For this review, take the finished solid that the model builds, in its own axes (mm). Face numbers are marked on the shaded views. Coordinates: 2 decimals unless noted, no trailing zeros. Loops run counter-clockwise (first coordinate to the right, second up) from the corner with the lowest first, then second, coordinate; pieces in that order, holes last. Notation, with made-up numbers: (78.5, 10) - (129.5, 10) arc R15 cw to (129.5, 22) - close; hole circle Ø7 at (27.5, -26.5). An arc over 180 degrees is marked (long way). One line per item, written item: value. Start each with the question number.
1. To check wall thickness, follow line 1 (Z direction, x = 157.5, y = 30.5) (3 decimals); line 2 (Z direction, x = 211, y = 21.5); line 3 (X direction, y = 26.5, z = -6). State the ranges of each line that lie inside material, in increasing order. Write a range as from..to.
2. The part is to be moulded in two halves that separate along X. For the marked faces 1, 2 and 3, say which applies: released by +X, released by -X, zero draft, split by the parting line, or undercut.
3. Take a section at C-C, the plane z = -21. State the section outline as (x, y) points, and give its area (3 significant figures).
4. Insertion check: pin 1 (12 mm diameter, centred on x = 223, y = 29.5, fed in from +Z); pin 2 (0.5 mm diameter, centred on y = 36.5, z = 1.5, fed in from +X); pin 3 (0.5 mm diameter, centred on y = 8, z = 1.5, fed in from -X). Each pin has a flat end and moves straight along its axis. Give the tip position at first contact, or say it passes through.
5. Take a section at B-B, the plane y = 15. State the section outline as (x, z) points (3 decimals).
6. Take a section at A-A, the plane x = 248. State the section outline as (y, z) points.
7. Take a section at D-D, the plane x = 177. State the section outline as (y, z) points (3 decimals).
```python
from build123d import *

# Parameters (mm, degrees)
BASE_FLANGE1_DEPTH = 44.45
SKETCH6_W          = 31.75
SKETCH6_H          = 3.429
CUT_EXTRUDE1_DEPTH = 284.468887342
SKETCH7_W          = 31.75
SKETCH7_H          = 3.429
CUT_EXTRUDE2_DEPTH = 272.141941158
FILLET1_R          = 12.7
CUT_EXTRUDE3_DEPTH = 284.468887342
CUT_EXTRUDE4_DEPTH = 272.141941158
SKETCH10_R         = 3.175
CUT_EXTRUDE5_DEPTH = 284.468887342


# Sheet-metal steps are written as plain solids
with BuildPart() as part:
    # Sketch1 → Base-Flange1 (new body)
    with BuildSketch(Plane(origin=(0, 0, 0), x_dir=(1, 0, 0), z_dir=(0, 1, 0))):
        with BuildLine():
            Line((0, 0), (193.606119446, 0))
            ThreePointArc((193.606119446, 0), (194.29331522, 0.075260177), (194.947932427, 0.297472776))
            Line((194.947932427, 0.297472776), (276.015713671, 38.1))
            Line((276.015713671, 38.1), (277.357526652, 35.222472776))
            Line((277.357526652, 35.222472776), (196.289745408, -2.580054448))
            ThreePointArc((196.289745408, -2.580054448), (194.980510995, -3.024479645), (193.606119446, -3.175))
            Line((193.606119446, -3.175), (0, -3.175))
            Line((0, -3.175), (0, 0))
        make_face()
    extrude(amount=BASE_FLANGE1_DEPTH)

    # Sketch6 → Cut-Extrude1 (cut, through all)
    with BuildSketch(Plane(origin=(0, 0, 0), x_dir=(-1, 0, 0), z_dir=(0, 0, -1))):
        with Locations((-136.525, 7.9375)):
            Rectangle(SKETCH6_W, SKETCH6_H)
        with Locations((-60.325, 36.5125)):
            Rectangle(SKETCH6_W, SKETCH6_H)
        with Locations((-136.525, 36.5125)):
            Rectangle(SKETCH6_W, SKETCH6_H)
        with Locations((-60.325, 7.9375)):
            Rectangle(SKETCH6_W, SKETCH6_H)
    extrude(amount=-CUT_EXTRUDE1_DEPTH, mode=Mode.SUBTRACT)

    # Sketch7 → Cut-Extrude2 (cut, through all)
    with BuildSketch(Plane(origin=(34.704969781, 0, 74.425047871), x_dir=(-0.9063077870366493, 0, 0.42261826174070083), z_dir=(-0.4226182617407009, 0, -0.9063077870366494))):
        with Locations((-228.156946417, 36.5125)):
            Rectangle(SKETCH7_W, SKETCH7_H)
        with Locations((-228.156946417, 7.9375)):
            Rectangle(SKETCH7_W, SKETCH7_H)
    extrude(amount=-CUT_EXTRUDE2_DEPTH, mode=Mode.SUBTRACT)

    # Fillet1
    fillet1_edges = [part.edges().sort_by_distance(p)[0] for p in [
        (0, 44.45, 1.5875),
        (0, 0, 1.5875),
        (276.686620162, 44.45, -36.661236388),
        (276.686620162, 0, -36.661236388),
    ]]
    fillet(fillet1_edges, radius=FILLET1_R)

    # Sketch8 → Cut-Extrude3 (cut, through all)
    with BuildSketch(Plane(origin=(0, 0, 0), x_dir=(-1, 0, 0), z_dir=(0, 0, -1))):
        with BuildLine():
            ThreePointArc((-44.938784585, 36.5125), (-46.030818439, 39.40175), (-47.122852293, 36.5125))
            ThreePointArc((-47.122852293, 36.5125), (-46.030818439, 33.62325), (-44.938784585, 36.5125))
        make_face()
        with BuildLine():
            ThreePointArc((-75.711215415, 36.5125), (-74.619181561, 33.62325), (-73.527147707, 36.5125))
            ThreePointArc((-73.527147707, 36.5125), (-74.619181561, 39.40175), (-75.711215415, 36.5125))
        make_face()
        with BuildLine():
            ThreePointArc((-121.138784585, 36.5125), (-122.230818439, 39.40175), (-123.322852293, 36.5125))
            ThreePointArc((-123.322852293, 36.5125), (-122.230818439, 33.62325), (-121.138784585, 36.5125))
        make_face()
        with BuildLine():
            ThreePointArc((-151.911215415, 36.5125), (-150.819181561, 33.62325), (-149.727147707, 36.5125))
            ThreePointArc((-149.727147707, 36.5125), (-150.819181561, 39.40175), (-151.911215415, 36.5125))
        make_face()
        with BuildLine():
            ThreePointArc((-151.911215415, 7.9375), (-150.819181561, 5.04825), (-149.727147707, 7.9375))
            ThreePointArc((-149.727147707, 7.9375), (-150.819181561, 10.82675), (-151.911215415, 7.9375))
        make_face()
        with BuildLine():
            ThreePointArc((-121.138784585, 7.9375), (-122.230818439, 10.82675), (-123.322852293, 7.9375))
            ThreePointArc((-123.322852293, 7.9375), (-122.230818439, 5.04825), (-121.138784585, 7.9375))
        make_face()
        with BuildLine():
            ThreePointArc((-75.711215415, 7.9375), (-74.619181561, 5.04825), (-73.527147707, 7.9375))
            ThreePointArc((-73.527147707, 7.9375), (-74.619181561, 10.82675), (-75.711215415, 7.9375))
        make_face()
        with BuildLine():
            ThreePointArc((-44.938784585, 7.9375), (-46.030818439, 10.82675), (-47.122852293, 7.9375))
            ThreePointArc((-47.122852293, 7.9375), (-46.030818439, 5.04825), (-44.938784585, 7.9375))
        make_face()
    extrude(amount=-CUT_EXTRUDE3_DEPTH, mode=Mode.SUBTRACT)

    # Sketch9 → Cut-Extrude4 (cut, through all)
    with BuildSketch(Plane(origin=(34.704969781, 0, 74.425047871), x_dir=(-0.9063077870366492, 0, 0.42261826174070116), z_dir=(-0.42261826174070116, 0, -0.9063077870366492))):
        with BuildLine():
            ThreePointArc((-214.95479871, 36.5125), (-213.862764856, 33.62325), (-212.770731003, 36.5125))
            ThreePointArc((-212.770731003, 36.5125), (-213.862764856, 39.40175), (-214.95479871, 36.5125))
        make_face()
        with BuildLine():
            ThreePointArc((-241.359094124, 36.5125), (-242.451127978, 39.40175), (-243.543161832, 36.5125))
            ThreePointArc((-243.543161832, 36.5125), (-242.451127978, 33.62325), (-241.359094124, 36.5125))
        make_face()
        with BuildLine():
            ThreePointArc((-241.359094124, 7.9375), (-242.451127978, 10.82675), (-243.543161832, 7.9375))
            ThreePointArc((-243.543161832, 7.9375), (-242.451127978, 5.04825), (-241.359094124, 7.9375))
        make_face()
        with BuildLine():
            ThreePointArc((-214.95479871, 7.9375), (-213.862764856, 5.04825), (-212.770731003, 7.9375))
            ThreePointArc((-212.770731003, 7.9375), (-213.862764856, 10.82675), (-214.95479871, 7.9375))
        make_face()
    extrude(amount=-CUT_EXTRUDE4_DEPTH, mode=Mode.SUBTRACT)

    # Sketch10 → Cut-Extrude5 (cut, through all)
    with BuildSketch(Plane(origin=(0, 0, 0), x_dir=(-1, 0, 0), z_dir=(0, 0, -1))):
        with Locations((-65.0875, 22.225)):
            Circle(SKETCH10_R)
    extrude(amount=-CUT_EXTRUDE5_DEPTH, mode=Mode.SUBTRACT)


solid = part.part
```
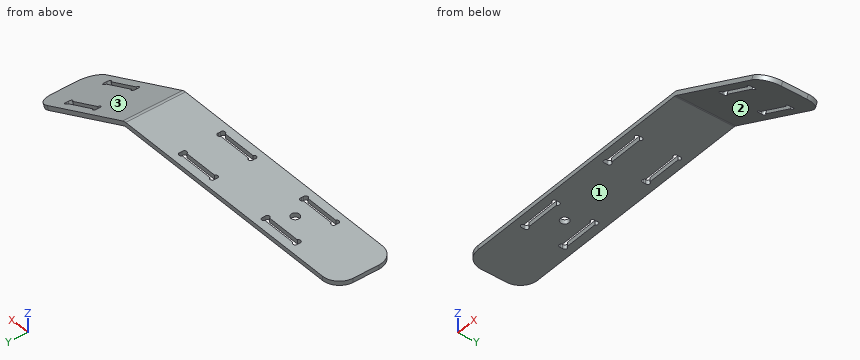
Solutions:
1. line 1: 0..3.175
1. line 2: -7.78..-4.28
1. line 3: 207.18..214.69
2. face 1: zero draft
2. face 2: released by -X
2. face 3: released by +X
3. outline: (239.34, 0) - (246.86, 0) - (246.86, 6.22) - (239.34, 6.22) - close; (239.34, 9.65) - (246.86, 9.65) - (246.86, 34.8) - (239.34, 34.8) - close; (239.34, 38.23) - (246.86, 38.23) - (246.86, 44.45) - (239.34, 44.45) - close
3. area: 282 mm2
4. pin 1: z = -7.08
4. pin 2: x = 199.14
4. pin 3: x = 0.81
5. outline: (0, 0) - (193.606, 0) arc R3.175 cw to (194.948, -0.297) - (276.016, -38.1) - (277.358, -35.222) - (196.29, 2.58) arc R6.35 ccw to (193.606, 3.175) - (0, 3.175) - close
6. outline: (0, -25.04) - (6.22, -25.04) - (6.22, -21.53) - (0, -21.53) - close; (9.65, -25.04) - (34.8, -25.04) - (34.8, -21.53) - (9.65, -21.53) - close; (38.23, -25.04) - (44.45, -25.04) - (44.45, -21.53) - (38.23, -21.53) - close
7. outline: (0, 0) - (44.45, 0) - (44.45, 3.175) - (0, 3.175) - close
